from build123d import *

# Parameters (mm, degrees)
SKETCH1_R          = 40
SKETCH1_W          = 80
SKETCH1_H          = 40
EXTRUDE1_DEPTH     = 20
SKETCH3_R          = 16
CUT_EXTRUDE1_DEPTH = 115.891252931
SKETCH7_R          = 7.5
CUT_EXTRUDE2_DEPTH = 115.891252931


with BuildPart() as part:
    # Sketch1 → Extrude1 (new body)
    with BuildSketch(Plane(origin=(0, 0, 0), x_dir=(1, 0, 0), z_dir=(0, 1, 0))):
        with Locations((40, 40)):
            Circle(SKETCH1_R)
        with Locations((40, 20)):
            Rectangle(SKETCH1_W, SKETCH1_H)
    extrude(amount=EXTRUDE1_DEPTH)

    # Sketch3 → Cut-Extrude1 (cut, through all)
    with BuildSketch(Plane(origin=(0, 20, 0), x_dir=(1, 0, 0), z_dir=(0, 1, 0))):
        with Locations(Location((40, 40, 0), (0, 0, 270))):
            Circle(SKETCH3_R)
    extrude(amount=-CUT_EXTRUDE1_DEPTH, mode=Mode.SUBTRACT)

    # Sketch7 → Cut-Extrude2 (cut, through all)
    with BuildSketch(Plane(origin=(0, 20, 0), x_dir=(1, 0, 0), z_dir=(0, 1, 0))):
        with Locations(Location((15, 15, 0), (0, 0, 270))):
            Circle(SKETCH7_R)
    cut_extrude2 = extrude(amount=-CUT_EXTRUDE2_DEPTH, mode=Mode.SUBTRACT)

    # Mirror1: Cut-Extrude2 across plane
    add(cut_extrude2.mirror(Plane(origin=(40, 0, 0), x_dir=(0, 0, 1), z_dir=(1, 0, 0))), mode=Mode.SUBTRACT)


solid = part.part
Model file for the job. Use its own axes, mm. Round coordinates to 2 decimals unless told otherwise and drop trailing zeros. Order: outer loops, then holes, each group sorted by start corner. A loop starts at its lowest first (then second) coordinate and runs counter-clockwise, first axis right, second up.
(1) Drill centre lines: line 1 (X direction, y = 6, z = -15); line 2 (X direction, y = 5.75, z = -10); line 3 (Z direction, x = 67.5, y = 10). Where is each one in solid material? Low to high.
(2) Band-saw the part on C-C (z = -9). List the corners of the cut face in (x, y).
(3) Pull direction Z, two halves, no side cores. Call faces 1 (the face through (59.9, 10.1, -20.5)), 2 (the face through (0, 10, -20)), 3 (the face through (39, 10, 0)): released by +Z, released by -Z, zero draft, split by the parting line, or undercut.
(4) Band-saw the part on A-A (x = 40). List the corners of the cut face in (y, z).
(5) Band-saw the part on B-B (y = 9.5). List the corners of the cut face in (x, z), then the cut area to 3 significant figures.
(6) Band-saw the part on D-D (z = -43.5). List the corners of the cut face in (x, y).
(7) Pin check, flat tips, straight feed: pin 1 (8 mm diameter, centred on x = 64, y = 10.5, fed in from -Z); pin 2 (5 mm diameter, centred on x = 25, y = 7, fed in from -Z); pin 3 (12 mm diameter, centred on x = 51.5, y = 5.5, fed in from -Z). Stop position of each tip, or through.
Verdict:
1. line 1: x = 0 to 7.5, 22.5 to 57.5, 72.5 to 80
1. line 2: x = 0 to 9.41, 20.59 to 59.41, 70.59 to 80
1. line 3: z = -69.05 to -22.07, -7.93 to 0
2. outline: (0, 0) - (10.5, 0) - (10.5, 20) - (0, 20) - close; (19.5, 0) - (60.5, 0) - (60.5, 20) - (19.5, 20) - close; (69.5, 0) - (80, 0) - (80, 20) - (69.5, 20) - close
3. face 1: undercut
3. face 2: zero draft
3. face 3: released by +Z
4. outline: (0, -80) - (20, -80) - (20, -56) - (0, -56) - close; (0, -24) - (20, -24) - (20, 0) - (0, 0) - close
5. outline: (0, -40) arc R40 ccw to (80, -40) - (80, 0) - (0, 0) - close; hole circle Ø15 at (15, -15); hole circle Ø32 at (40, -40); hole circle Ø15 at (65, -15)
5. area: 4,560 mm2
6. outline: (0.15, 0) - (24.39, 0) - (24.39, 20) - (0.15, 20) - close; (55.61, 0) - (79.85, 0) - (79.85, 20) - (55.61, 20) - close
7. pin 1: stops at z = -74.64
7. pin 2: stops at z = -78
7. pin 3: stops at z = -79.62
